Model file for the job. Use its own axes, mm. Face numbers are marked on the shaded views. A direction names the side the tool comes from. Round coordinates to 2 decimals unless told otherwise and drop trailing zeros. Order: outer loops, then holes, each group sorted by start corner. A loop starts at its lowest first (then second) coordinate and runs counter-clockwise, first axis right, second up. Notation, with made-up numbers: (81.25, 25.5) - (93.25, 25.5) arc R21 ccw to (93.25, 29.5) - close; hole circle Ø5 at (32, -28). An arc over 180 degrees is marked (long way). Put each result on its own line as item: value. Start each with the question number.
Item 1: Pin check, flat tips, straight feed: pin 1 Ø5 at (x, y) = (-65.5, 4) entering from -Z; pin 2 Ø3.5 at (y, z) = (5.5, 1.5) entering from +X; pin 3 Ø2 at (x, y) = (10.5, 2.5) entering from +Z. Stop position of each tip, or through.
Item 2: Saw through at D-D on x = -5.5. List the corners of the cut face in (y, z), plus the area to 3 significant figures.
Item 3: Saw through at A-A on x = -59.5. List the corners of the cut face in (y, z), plus the area to 4 significant figures.
Item 4: Saw through at B-B on z = 4.5. List the corners of the cut face in (x, y).
Item 5: Saw through at C-C on z = -22. List the corners of the cut face in (x, y).
Item 6: Probe probe 1 along X at (y, z) = (4.5, 30); probe 2 along X at (y, z) = (6.25, 8); probe 3 along Y at (x, z) = (22.5, 9.5). List the from-to ranges inside material, lowest first.
Item 7: Which spindle directions (+Z, -Z, +X, -X, +Y, -Y) get a long thin tool onto all of the face, cutting with end or side? Do the marked faces 5, 6 and 7. Say none if no direction does.
Item 8: Mould opens along Z. For the marked faces 1, 2, 3 and 4 say: pulls with the +Z half, pulls with the -Z half, needs draft (parallel to the pull), parting line crosses it, or undercut.
```python
from build123d import *

# Parameters (mm, degrees)
SKETCH1_W           = 89
SKETCH1_H           = 70
SKETCH1_R           = 1
BOSS_EXTRUDE1_DEPTH = 10
CUT_EXTRUDE2_DEPTH  = 7
SKETCH6_W           = 30
SKETCH6_H           = 41.5
SKETCH6_R           = 1.25
BOSS_EXTRUDE2_DEPTH = 10
SKETCH7_W           = 34
SKETCH7_H           = 13.5
CUT_EXTRUDE3_DEPTH  = 7


with BuildPart() as part:
    # Sketch1 → Boss-Extrude1 (new body)
    with BuildSketch(Plane(origin=(0, 0, 0), x_dir=(1, 0, 0), z_dir=(0, 1, 0))):
        Rectangle(SKETCH1_W, SKETCH1_H)
        with Locations(Location((-39.5, 30, 0), (0, 0, 270))):
            Circle(SKETCH1_R, mode=Mode.SUBTRACT)
        with Locations(Location((39.5, 30, 0), (0, 0, 90))):
            Circle(SKETCH1_R, mode=Mode.SUBTRACT)
        with Locations(Location((39.5, -30, 0), (0, 0, 270))):
            Circle(SKETCH1_R, mode=Mode.SUBTRACT)
        with Locations(Location((-39.5, -30, 0), (0, 0, 90))):
            Circle(SKETCH1_R, mode=Mode.SUBTRACT)
    extrude(amount=BOSS_EXTRUDE1_DEPTH)

    # Sketch3 → Cut-Extrude2 (cut)
    with BuildSketch(Plane(origin=(0, 10, 0), x_dir=(1, 0, 0), z_dir=(0, 1, 0))):
        Polygon((-44.5, -20), (-29.5, -35), (29.5, -35), (44.5, -20), (44.5, 20), (29.5, 35), (-29.5, 35), (-44.5, 20), align=None)
    extrude(amount=-CUT_EXTRUDE2_DEPTH, mode=Mode.SUBTRACT)

    # Sketch6 → Boss-Extrude2 (add)
    with BuildSketch(Plane.XZ):
        with Locations((-59.5, 17.25)):
            Rectangle(SKETCH6_W, SKETCH6_H)
        with Locations(Location((-59.5, 30, 0), (0, 0, 270))):
            Circle(SKETCH6_R, mode=Mode.SUBTRACT)
        with Locations(Location((-59.5, 4.5, 0), (0, 0, 270))):
            Circle(SKETCH6_R, mode=Mode.SUBTRACT)
    extrude(amount=-BOSS_EXTRUDE2_DEPTH)

    # Sketch7 → Cut-Extrude3 (cut)
    with BuildSketch(Plane(origin=(0, 10, 0), x_dir=(1, 0, 0), z_dir=(0, 1, 0))):
        with Locations((-57.5, -17.25)):
            Rectangle(SKETCH7_W, SKETCH7_H)
    extrude(amount=-CUT_EXTRUDE3_DEPTH, mode=Mode.SUBTRACT)


solid = part.part
```
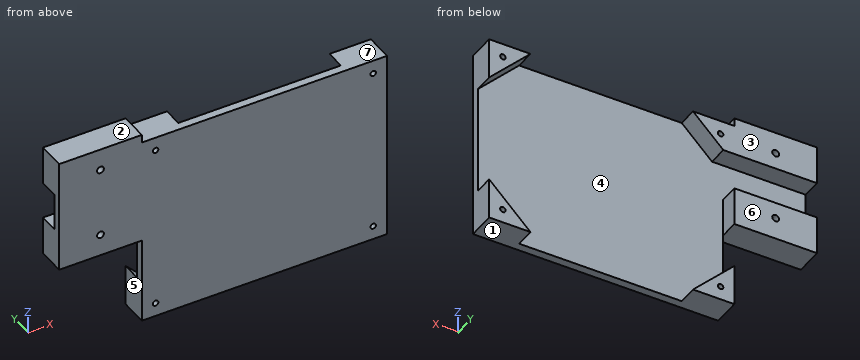
Results found:
1. pin 1: stops at z = -3.5
1. pin 2: stops at x = -44.5
1. pin 3: stops at z = 35
2. outline: (0, -35) - (3, -35) - (3, 35) - (0, 35) - close
2. area: 210 mm²
3. outline: (0, -3.5) - (10, -3.5) - (10, 3.25) - (0, 3.25) - close; (0, 5.75) - (10, 5.75) - (10, 10.5) - (3, 10.5) - (3, 24) - (10, 24) - (10, 28.75) - (0, 28.75) - close; (0, 31.25) - (10, 31.25) - (10, 38) - (0, 38) - close
3. area: 270.5 mm²
4. outline: (-74.5, 0) - (-60.75, 0) - (-60.75, 10) - (-74.5, 10) - close; (-58.25, 0) - (44.5, 0) - (44.5, 3) - (-44.5, 3) - (-44.5, 10) - (-58.25, 10) - close
5. outline: (-44.5, 0) - (44.5, 0) - (44.5, 10) - (42.5, 10) - (42.5, 3) - (-42.5, 3) - (-42.5, 10) - (-44.5, 10) - close
6. probe 1: x = -74.5 to -60.75, -58.25 to -40.5, -38.5 to -34.5, 34.5 to 38.5, 40.5 to 44.5
6. probe 2: x = -74.5 to -44.5
6. probe 3: y = 0 to 3
7. face 5: -Z, -X, +Y, -Y
7. face 6: +Z, -Z, +X, -X, +Y
7. face 7: +Z, +X, +Y, -Y
8. face 1: pulls with the -Z half
8. face 2: pulls with the +Z half
8. face 3: needs draft
8. face 4: undercut
